```python
from build123d import *

# Parameters (mm, degrees)
CROQUIS1_W              = 61
CROQUIS1_H              = 100
SALIENTE_EXTRUIR1_DEPTH = 3
SALIENTE_EXTRUIR4_DEPTH = 3
CROQUIS19_W             = 61
CROQUIS19_H             = 5.5
CORTAR_EXTRUIR11_DEPTH  = 10
CORTAR_EXTRUIR7_DEPTH   = 4
REDONDEO3_R             = 2
CROQUIS15_R             = 1.6
CORTAR_EXTRUIR8_DEPTH   = 4.0000001
CROQUIS16_R             = 3
CORTAR_EXTRUIR9_DEPTH   = 4.0000001
CROQUIS17_W             = 3.1
CROQUIS17_H             = 10.1
CORTAR_EXTRUIR10_DEPTH  = 10
CORTAR_EXTRUIR13_DEPTH  = 4.0000001
CROQUIS20_W             = 10.1
CROQUIS20_H             = 3.1
CORTAR_EXTRUIR12_DEPTH  = 10
CROQUIS22_R             = 2
CORTAR_EXTRUIR14_DEPTH  = 10


with BuildPart() as part:
    # Croquis1 → Saliente-Extruir1 (new body)
    with BuildSketch(Plane(origin=(0, 0, 0), x_dir=(1, 0, 0), z_dir=(0, 1, 0))):
        with Locations((0, -18)):
            Rectangle(CROQUIS1_W, CROQUIS1_H)
    extrude(amount=SALIENTE_EXTRUIR1_DEPTH)

    # Croquis7 → Saliente-Extruir4 (add, through all)
    with BuildSketch(Plane(origin=(0, 3, 0), x_dir=(1, 0, 0), z_dir=(0, 1, 0))):
        with BuildLine():
            Line((-50, -62.5), (-50, 32))
            ThreePointArc((-50, 32), (0, 44.950013881), (50, 32))
            Line((50, 32), (50, -62.5))
            Line((50, -62.5), (-50, -62.5))
        make_face()
    extrude(amount=-SALIENTE_EXTRUIR4_DEPTH)

    # Croquis19 → Cortar-Extruir11 (cut)
    with BuildSketch(Plane(origin=(0, 3, 0), x_dir=(1, 0, 0), z_dir=(0, 1, 0))):
        with Locations((0, -65.25)):
            Rectangle(CROQUIS19_W, CROQUIS19_H)
    extrude(amount=-CORTAR_EXTRUIR11_DEPTH, mode=Mode.SUBTRACT)

    # Croquis14 → Cortar-Extruir7 (cut, through all)
    with BuildSketch(Plane(origin=(0, 3, 0), x_dir=(1, 0, 0), z_dir=(0, 1, 0))):
        with BuildLine():
            Line((-50, -24), (-50, -62.5))
            Line((-50, -62.5), (-28, -62.5))
            add(Edge.make_bspline(
                [(-50, -24), (-50, -36), (-40, -62.5), (-28, -62.5)],
                knots=[0, 0, 0, 0, 1, 1, 1, 1], degree=3))
        make_face()
    cortar_extruir7 = extrude(amount=-CORTAR_EXTRUIR7_DEPTH, mode=Mode.SUBTRACT)

    # Redondeo3
    redondeo3_edges = [part.edges().sort_by_distance(p)[0] for p in [
        (-50, 1.5, -32),
        (50, 1.5, -32),
    ]]
    fillet(redondeo3_edges, radius=REDONDEO3_R)

    # Croquis15 → Cortar-Extruir8 (cut, through all)
    with BuildSketch(Plane(origin=(0, 3, 0), x_dir=(1, 0, 0), z_dir=(0, 1, 0))):
        with Locations((-19.5, 14)):
            Circle(CROQUIS15_R)
        with Locations((19.5, 14)):
            Circle(CROQUIS15_R)
        with Locations((-19.5, -50)):
            Circle(CROQUIS15_R)
        with Locations((19.5, -50)):
            Circle(CROQUIS15_R)
    extrude(amount=-CORTAR_EXTRUIR8_DEPTH, mode=Mode.SUBTRACT)

    # Croquis16 → Cortar-Extruir9 (cut, through all)
    with BuildSketch(Plane(origin=(0, 3, 0), x_dir=(1, 0, 0), z_dir=(0, 1, 0))):
        with Locations((0, -16.75)):
            Circle(CROQUIS16_R)
    extrude(amount=-CORTAR_EXTRUIR9_DEPTH, mode=Mode.SUBTRACT)

    # Croquis17 → Cortar-Extruir10 (cut)
    with BuildSketch(Plane(origin=(0, 3, 0), x_dir=(1, 0, 0), z_dir=(0, 1, 0))):
        with Locations((-44.5, 20.395080133)):
            Rectangle(CROQUIS17_W, CROQUIS17_H)
        with Locations((-44.5, 0.395080133)):
            Rectangle(CROQUIS17_W, CROQUIS17_H)
        with Locations((-44.5, -19.604919867)):
            Rectangle(CROQUIS17_W, CROQUIS17_H)
    cortar_extruir10 = extrude(amount=-CORTAR_EXTRUIR10_DEPTH, mode=Mode.SUBTRACT)

    # Croquis21 → Cortar-Extruir13 (cut, through all)
    with BuildSketch(Plane(origin=(0, 3, 0), x_dir=(1, 0, 0), z_dir=(0, 1, 0))):
        Polygon((-44.645093952, -37.058907452), (-42.934664747, -41.863533549), (-40.014205747, -40.823860895), (-41.724634952, -36.019234798), align=None)
        Polygon((-38.866197007, -50.280851683), (-35.970669214, -54.479175015), (-33.418747189, -52.719148317), (-36.314274981, -48.520824985), align=None)
    cortar_extruir13 = extrude(amount=-CORTAR_EXTRUIR13_DEPTH, mode=Mode.SUBTRACT)

    # Simetría1: Cortar-Extruir7, Cortar-Extruir10, Cortar-Extruir13 across plane
    add(cortar_extruir7.mirror(Plane(origin=(0, 0, 0), x_dir=(0, 0, 1), z_dir=(1, 0, 0))), mode=Mode.SUBTRACT)
    add(cortar_extruir10.mirror(Plane(origin=(0, 0, 0), x_dir=(0, 0, 1), z_dir=(1, 0, 0))), mode=Mode.SUBTRACT)
    add(cortar_extruir13.mirror(Plane(origin=(0, 0, 0), x_dir=(0, 0, 1), z_dir=(1, 0, 0))), mode=Mode.SUBTRACT)

    # Croquis20 → Cortar-Extruir12 (cut)
    with BuildSketch(Plane(origin=(0, 3, 0), x_dir=(1, 0, 0), z_dir=(0, 1, 0))):
        with Locations((0, -58.5)):
            Rectangle(CROQUIS20_W, CROQUIS20_H)
        with Locations((20, -58.5)):
            Rectangle(CROQUIS20_W, CROQUIS20_H)
        with Locations((-20, -58.5)):
            Rectangle(CROQUIS20_W, CROQUIS20_H)
    extrude(amount=-CORTAR_EXTRUIR12_DEPTH, mode=Mode.SUBTRACT)

    # Croquis22 → Cortar-Extruir14 (cut)
    with BuildSketch(Plane(origin=(0, 3, 0), x_dir=(1, 0, 0), z_dir=(0, 1, 0))):
        with Locations((-20.25, -35)):
            Circle(CROQUIS22_R)
    extrude(amount=-CORTAR_EXTRUIR14_DEPTH, mode=Mode.SUBTRACT)


solid = part.part
```
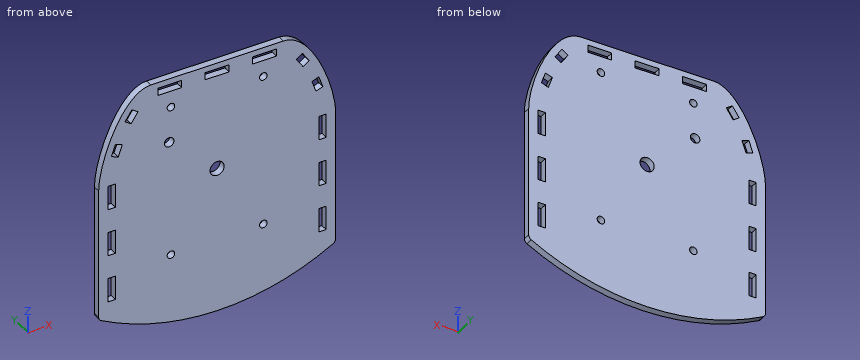
Work out the finished part from the listing and answer in its coordinate system (mm). Coordinates: 2 decimals unless noted, no trailing zeros. Loops run counter-clockwise (first coordinate to the right, second up) from the corner with the lowest first, then second, coordinate; pieces in that order, holes last.
1) Section B-B (x = 0) is taken. Give the vertices of the cut face in (y, z).
Results:
outline: (0, -44.95) - (3, -44.95) - (3, 13.75) - (0, 13.75) - close; (0, 19.75) - (3, 19.75) - (3, 56.95) - (0, 56.95) - close; (0, 60.05) - (3, 60.05) - (3, 62.5) - (0, 62.5) - close
2) Flat-ended cylindrical pins translate along their axes: pin 1 (0.9 mm diameter, centred on x = -44.5, y = 2, fed in from +Z); pin 2 (0.9 mm diameter, centred on y = 1.5, z = 59, fed in from -X). Find the tip coordinate at first contact, or state that the pin passes through.
Results:
pin 1: stops at z = 46.6
pin 2: stops at x = -36.12
3) Section A-A (z = -14) is taken. Give the vertices of the cut face in (x, y).
Results:
outline: (-50, 0) - (-21.1, 0) - (-21.1, 3) - (-50, 3) - close; (-17.9, 0) - (17.9, 0) - (17.9, 3) - (-17.9, 3) - close; (21.1, 0) - (50, 0) - (50, 3) - (21.1, 3) - close
4) Section C-C (y = 1.55) is taken. Give the number of separate pieces and of enclosed holes in the cut face, plus the area to 3 significant figures.
Results:
separate pieces: 1
enclosed holes: 19
area: 9,450 mm2
5) Consider probe 1 along X at (y, z) = (0.45, -1.5); probe 2 along X at (y, z) = (0.7, -14); probe 3 along Z at (x, y) = (-22, 0.3). Determine where each line is inside the solid, lowest interval first.
Results:
probe 1: x = -50 to -46.05, -42.95 to 42.95, 46.05 to 50
probe 2: x = -50 to -21.1, -17.9 to 17.9, 21.1 to 50
probe 3: z = -42.57 to 34.03, 35.97 to 56.95, 60.05 to 62.5
